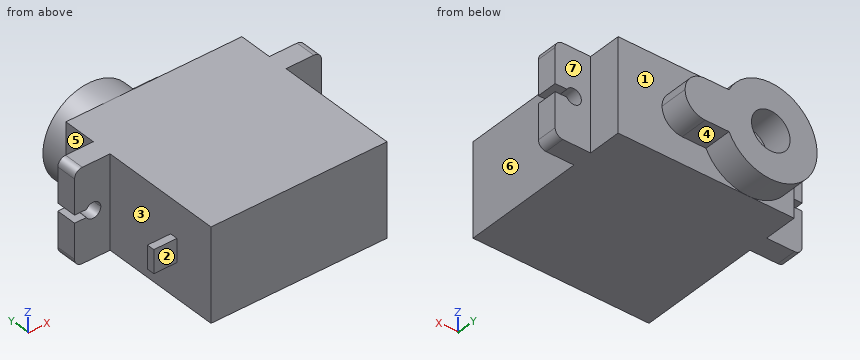
from build123d import *

# Parameters (mm, degrees)
SKETCH1_W                       = 22.8
SKETCH1_H                       = 12
BOSS_EXTRUDE1_DEPTH             = 16
SKETCH2_W                       = 32
SKETCH2_H                       = 12
BOSS_EXTRUDE2_DEPTH             = 2.65
BOSS_EXTRUDE3_REACH             = 25.409
SKETCH3_W                       = 22.8
SKETCH3_H                       = 23
BOSS_EXTRUDE3_DIRECTION_2_REACH = 25.409
CUT_EXTRUDE1_REACH              = 27.295
FILLET1_R                       = 1
SKETCH5_R                       = 6
BOSS_EXTRUDE4_DEPTH             = 3.65
BOSS_EXTRUDE5_DEPTH             = 3.65
SKETCH7_R                       = 2.5
CUT_EXTRUDE2_DEPTH              = 3.65
SKETCH8_W                       = 3
SKETCH8_H                       = 1
BOSS_EXTRUDE6_DEPTH             = 3


with BuildPart() as part:
    # Sketch1 → Boss-Extrude1 (new body)
    with BuildSketch(Plane(origin=(0, 0, 0), x_dir=(1, 0, 0), z_dir=(0, 1, 0))):
        Rectangle(SKETCH1_W, SKETCH1_H)
    extrude(amount=-BOSS_EXTRUDE1_DEPTH)

    # Sketch2 → Boss-Extrude2 (add)
    with BuildSketch(Plane(origin=(0, 0, 0), x_dir=(1, 0, 0), z_dir=(0, 1, 0))):
        Rectangle(SKETCH2_W, SKETCH2_H)
    extrude(amount=BOSS_EXTRUDE2_DEPTH)

    # Boss-Extrude3: up to this face of the body (flat: up to its plane)
    boss_extrude3_end = Plane(part.part.faces().sort_by_distance((0, -6.241192171, 6))[0])
    # Sketch3 → Boss-Extrude3 (add, up to the picked face)
    with BuildSketch(Plane.XY, mode=Mode.PRIVATE) as boss_extrude3_sk1:
        with Locations((0, -4.5)):
            Rectangle(SKETCH3_W, SKETCH3_H)
    boss_extrude3_tool1 = split(extrude(boss_extrude3_sk1.sketch, amount=BOSS_EXTRUDE3_REACH, mode=Mode.PRIVATE), bisect_by=boss_extrude3_end, keep=Keep.BOTH, mode=Mode.PRIVATE)
    add(boss_extrude3_tool1.solids().sort_by(Axis((0, -4.5, 0), (0, 0, 1)))[0])

    # Boss-Extrude3 direction 2: up to this face of the body (flat: up to its plane)
    boss_extrude3_direction_2_end = Plane(part.part.faces().sort_by_distance((0, -6.241192171, -6))[0])
    # Sketch3 → Boss-Extrude3 direction 2 (add, up to the picked face)
    with BuildSketch(Plane.XY, mode=Mode.PRIVATE) as boss_extrude3_direction_2_sk1:
        with Locations((0, -4.5)):
            Rectangle(SKETCH3_W, SKETCH3_H)
    boss_extrude3_direction_2_tool1 = split(extrude(boss_extrude3_direction_2_sk1.sketch, amount=-BOSS_EXTRUDE3_DIRECTION_2_REACH, mode=Mode.PRIVATE), bisect_by=boss_extrude3_direction_2_end, keep=Keep.BOTH, mode=Mode.PRIVATE)
    add(boss_extrude3_direction_2_tool1.solids().sort_by(Axis((0, -4.5, 0), (0, 0, -1)))[0])

    # Sketch4 → Cut-Extrude1 (cut, up to next)
    with BuildSketch(Plane(origin=(0, 2.65, 0), x_dir=(1, 0, 0), z_dir=(0, 1, 0)), mode=Mode.PRIVATE) as cut_extrude1_sk1:
        with BuildLine():
            ThreePointArc((14.6, 0), (14.565925826, 0.258819045), (14.466025404, 0.5))
            Line((14.466025404, 0.5), (13.6, 0.5))
            Line((13.6, 0.5), (13.6, -0.5))
            Line((13.6, -0.5), (14.466025404, -0.5))
            ThreePointArc((14.466025404, -0.5), (14.565925826, -0.258819045), (14.6, 0))
        make_face()
    cut_extrude1_tool1 = extrude(cut_extrude1_sk1.sketch, amount=-CUT_EXTRUDE1_REACH, mode=Mode.PRIVATE) & part.part
    # Sketch4 → Cut-Extrude1 (cut, up to next)
    with BuildSketch(Plane(origin=(0, 2.65, 0), x_dir=(1, 0, 0), z_dir=(0, 1, 0)), mode=Mode.PRIVATE) as cut_extrude1_sk2:
        with BuildLine():
            Line((13.6, 0.5), (14.466025404, 0.5))
            ThreePointArc((14.466025404, 0.5), (12.6, 0), (14.466025404, -0.5))
            Line((14.466025404, -0.5), (13.6, -0.5))
            Line((13.6, -0.5), (13.6, 0.5))
        make_face()
    cut_extrude1_tool2 = extrude(cut_extrude1_sk2.sketch, amount=-CUT_EXTRUDE1_REACH, mode=Mode.PRIVATE) & part.part
    # Sketch4 → Cut-Extrude1 (cut, up to next)
    with BuildSketch(Plane(origin=(0, 2.65, 0), x_dir=(1, 0, 0), z_dir=(0, 1, 0)), mode=Mode.PRIVATE) as cut_extrude1_sk3:
        with BuildLine():
            ThreePointArc((14.6, 0), (14.565925826, 0.258819045), (14.466025404, 0.5))
            Line((14.466025404, 0.5), (13.6, 0.5))
            Line((13.6, 0.5), (13.6, -0.5))
            Line((13.6, -0.5), (14.466025404, -0.5))
            ThreePointArc((14.466025404, -0.5), (14.565925826, -0.258819045), (14.6, 0))
        make_face()
    cut_extrude1_tool3 = extrude(cut_extrude1_sk3.sketch, amount=-CUT_EXTRUDE1_REACH, mode=Mode.PRIVATE) & part.part
    # Sketch4 → Cut-Extrude1 (cut, up to next)
    with BuildSketch(Plane(origin=(0, 2.65, 0), x_dir=(1, 0, 0), z_dir=(0, 1, 0)), mode=Mode.PRIVATE) as cut_extrude1_sk4:
        with BuildLine():
            Line((13.6, 0.5), (14.466025404, 0.5))
            ThreePointArc((14.466025404, 0.5), (12.6, 0), (14.466025404, -0.5))
            Line((14.466025404, -0.5), (13.6, -0.5))
            Line((13.6, -0.5), (13.6, 0.5))
        make_face()
    cut_extrude1_tool4 = extrude(cut_extrude1_sk4.sketch, amount=-CUT_EXTRUDE1_REACH, mode=Mode.PRIVATE) & part.part
    # Sketch4 → Cut-Extrude1 (cut, up to next)
    with BuildSketch(Plane(origin=(0, 2.65, 0), x_dir=(1, 0, 0), z_dir=(0, 1, 0)), mode=Mode.PRIVATE) as cut_extrude1_sk5:
        with BuildLine():
            Line((16, -0.5), (16, 0.5))
            Line((16, 0.5), (14.466025404, 0.5))
            ThreePointArc((14.466025404, 0.5), (14.565925826, 0.258819045), (14.6, 0))
            ThreePointArc((14.6, 0), (14.565925826, -0.258819045), (14.466025404, -0.5))
            Line((14.466025404, -0.5), (16, -0.5))
        make_face()
    cut_extrude1_tool5 = extrude(cut_extrude1_sk5.sketch, amount=-CUT_EXTRUDE1_REACH, mode=Mode.PRIVATE) & part.part
    # Sketch4 → Cut-Extrude1 (cut, up to next)
    with BuildSketch(Plane(origin=(0, 2.65, 0), x_dir=(1, 0, 0), z_dir=(0, 1, 0)), mode=Mode.PRIVATE) as cut_extrude1_sk6:
        with BuildLine():
            Line((-14.466025404, 0.5), (-16, 0.5))
            Line((-16, 0.5), (-16, -0.5))
            Line((-16, -0.5), (-14.466025404, -0.5))
            ThreePointArc((-14.466025404, -0.5), (-14.6, 0), (-14.466025404, 0.5))
        make_face()
    cut_extrude1_tool6 = extrude(cut_extrude1_sk6.sketch, amount=-CUT_EXTRUDE1_REACH, mode=Mode.PRIVATE) & part.part
    # Sketch4 → Cut-Extrude1 (cut, up to next)
    with BuildSketch(Plane(origin=(0, 2.65, 0), x_dir=(1, 0, 0), z_dir=(0, 1, 0)), mode=Mode.PRIVATE) as cut_extrude1_sk7:
        with BuildLine():
            ThreePointArc((-12.6, 0), (-13.341180955, 0.965925826), (-14.466025404, 0.5))
            Line((-14.466025404, 0.5), (-13.6, 0.5))
            Line((-13.6, 0.5), (-13.6, -0.5))
            Line((-13.6, -0.5), (-14.466025404, -0.5))
            ThreePointArc((-14.466025404, -0.5), (-13.341180955, -0.965925826), (-12.6, 0))
        make_face()
    cut_extrude1_tool7 = extrude(cut_extrude1_sk7.sketch, amount=-CUT_EXTRUDE1_REACH, mode=Mode.PRIVATE) & part.part
    # Sketch4 → Cut-Extrude1 (cut, up to next)
    with BuildSketch(Plane(origin=(0, 2.65, 0), x_dir=(1, 0, 0), z_dir=(0, 1, 0)), mode=Mode.PRIVATE) as cut_extrude1_sk8:
        with BuildLine():
            Line((-13.6, 0.5), (-14.466025404, 0.5))
            ThreePointArc((-14.466025404, 0.5), (-14.6, 0), (-14.466025404, -0.5))
            Line((-14.466025404, -0.5), (-13.6, -0.5))
            Line((-13.6, -0.5), (-13.6, 0.5))
        make_face()
    cut_extrude1_tool8 = extrude(cut_extrude1_sk8.sketch, amount=-CUT_EXTRUDE1_REACH, mode=Mode.PRIVATE) & part.part
    # Sketch4 → Cut-Extrude1 (cut, up to next)
    with BuildSketch(Plane(origin=(0, 2.65, 0), x_dir=(1, 0, 0), z_dir=(0, 1, 0)), mode=Mode.PRIVATE) as cut_extrude1_sk9:
        with BuildLine():
            ThreePointArc((-12.6, 0), (-13.341180955, 0.965925826), (-14.466025404, 0.5))
            Line((-14.466025404, 0.5), (-13.6, 0.5))
            Line((-13.6, 0.5), (-13.6, -0.5))
            Line((-13.6, -0.5), (-14.466025404, -0.5))
            ThreePointArc((-14.466025404, -0.5), (-13.341180955, -0.965925826), (-12.6, 0))
        make_face()
    cut_extrude1_tool9 = extrude(cut_extrude1_sk9.sketch, amount=-CUT_EXTRUDE1_REACH, mode=Mode.PRIVATE) & part.part
    # Sketch4 → Cut-Extrude1 (cut, up to next)
    with BuildSketch(Plane(origin=(0, 2.65, 0), x_dir=(1, 0, 0), z_dir=(0, 1, 0)), mode=Mode.PRIVATE) as cut_extrude1_sk10:
        with BuildLine():
            Line((-13.6, 0.5), (-14.466025404, 0.5))
            ThreePointArc((-14.466025404, 0.5), (-14.6, 0), (-14.466025404, -0.5))
            Line((-14.466025404, -0.5), (-13.6, -0.5))
            Line((-13.6, -0.5), (-13.6, 0.5))
        make_face()
    cut_extrude1_tool10 = extrude(cut_extrude1_sk10.sketch, amount=-CUT_EXTRUDE1_REACH, mode=Mode.PRIVATE) & part.part
    add(cut_extrude1_tool1.solids().sort_by_distance((14.079122, 2.65, 0))[0], mode=Mode.SUBTRACT)
    add(cut_extrude1_tool2.solids().sort_by_distance((13.390235, 2.65, 0))[0], mode=Mode.SUBTRACT)
    add(cut_extrude1_tool3.solids().sort_by_distance((14.079122, 2.65, 0))[0], mode=Mode.SUBTRACT)
    add(cut_extrude1_tool4.solids().sort_by_distance((13.390235, 2.65, 0))[0], mode=Mode.SUBTRACT)
    add(cut_extrude1_tool5.solids().sort_by_distance((15.277765, 2.65, 0))[0], mode=Mode.SUBTRACT)
    add(cut_extrude1_tool6.solids().sort_by_distance((-15.277765, 2.65, 0))[0], mode=Mode.SUBTRACT)
    add(cut_extrude1_tool7.solids().sort_by_distance((-13.390235, 2.65, 0))[0], mode=Mode.SUBTRACT)
    add(cut_extrude1_tool8.solids().sort_by_distance((-14.079122, 2.65, 0))[0], mode=Mode.SUBTRACT)
    add(cut_extrude1_tool9.solids().sort_by_distance((-13.390235, 2.65, 0))[0], mode=Mode.SUBTRACT)
    add(cut_extrude1_tool10.solids().sort_by_distance((-14.079122, 2.65, 0))[0], mode=Mode.SUBTRACT)

    # Fillet1
    fillet1_edges = [part.edges().sort_by_distance(p)[0] for p in [
        (16, 1.325, 6),
        (16, 1.325, -6),
        (-16, 1.325, -6),
        (-16, 1.325, 6),
    ]]
    fillet(fillet1_edges, radius=FILLET1_R)

    # Sketch5 → Boss-Extrude4 (add)
    with BuildSketch(Plane(origin=(0, 7, 0), x_dir=(1, 0, 0), z_dir=(0, 1, 0))):
        with Locations(Location((-5.4, 0, 0), (0, 0, 270))):
            Circle(SKETCH5_R)
    extrude(amount=BOSS_EXTRUDE4_DEPTH)

    # Sketch6 → Boss-Extrude5 (add)
    with BuildSketch(Plane(origin=(0, 7, 0), x_dir=(1, 0, 0), z_dir=(0, 1, 0))):
        with BuildLine():
            Line((0.007402334, -2.6), (3.1, -2.6))
            ThreePointArc((3.1, -2.6), (1.487245955, -2.039368625), (0.57, -0.599249531))
            ThreePointArc((0.57, -0.599249531), (0.375990961, -1.624170072), (0.007402334, -2.6))
        make_face()
        with BuildLine():
            ThreePointArc((0.57, 0.599249531), (1.487245955, 2.039368625), (3.1, 2.6))
            Line((3.1, 2.6), (0.007402334, 2.6))
            ThreePointArc((0.007402334, 2.6), (0.375990961, 1.624170072), (0.57, 0.599249531))
        make_face()
        with BuildLine():
            ThreePointArc((5.7, 0), (4.938477631, 1.838477631), (3.1, 2.6))
            ThreePointArc((3.1, 2.6), (1.487245955, 2.039368625), (0.57, 0.599249531))
            ThreePointArc((0.57, 0.599249531), (0.592495307, 0.3), (0.6, 0))
            ThreePointArc((0.6, 0), (0.592495307, -0.3), (0.57, -0.599249531))
            ThreePointArc((0.57, -0.599249531), (1.487245955, -2.039368625), (3.1, -2.6))
            ThreePointArc((3.1, -2.6), (4.938477631, -1.838477631), (5.7, 0))
        make_face()
        with BuildLine():
            ThreePointArc((0.6, 0), (0.592495307, 0.3), (0.57, 0.599249531))
            ThreePointArc((0.57, 0.599249531), (0.5, 0), (0.57, -0.599249531))
            ThreePointArc((0.57, -0.599249531), (0.592495307, -0.3), (0.6, 0))
        make_face()
    extrude(amount=BOSS_EXTRUDE5_DEPTH)

    # Sketch7 → Cut-Extrude2 (cut)
    with BuildSketch(Plane(origin=(0, 10.65, 0), x_dir=(1, 0, 0), z_dir=(0, 1, 0))):
        with Locations(Location((-5.4, 0, 0), (0, 0, 270))):
            Circle(SKETCH7_R)
    extrude(amount=-CUT_EXTRUDE2_DEPTH, mode=Mode.SUBTRACT)

    # Sketch8 → Boss-Extrude6 (add)
    with BuildSketch(Plane.ZY.offset(11.4)):
        with Locations((0, -10.1)):
            Rectangle(SKETCH8_W, SKETCH8_H)
    extrude(amount=BOSS_EXTRUDE6_DEPTH)


solid = part.part
Geometry check sheet. Reference: the model listing, model coordinates, mm. Face numbers are marked on the shaded views. A direction names the side the tool comes from. Round coordinates to 2 decimals unless told otherwise and drop trailing zeros. Order: outer loops, then holes, each group sorted by start corner. A loop starts at its lowest first (then second) coordinate and runs counter-clockwise, first axis right, second up. Notation, with made-up numbers: (10, 61) - (40, 61) arc R32 ccw to (40, 93) - close; hole circle Ø6 at (69, -12). An arc over 180 degrees is marked (long way). One line per question, with ' | ' between items. Start each with the question number.
(1) Depth check by flat-ended pin: pin 1 Ø3 at (x, z) = (-5.4, 0) entering from +Y; pin 2 Ø3.5 at (x, z) = (13.5, 1.5) entering from +Y; pin 3 Ø1.5 at (y, z) = (3.5, -2) entering from -X. Enter the tip coordinate at first touch or a pass-through.
(2) Sectioned sample at D-D on x = 4. Record the cut outline in (y, z).
(3) Access from +Z, -Z, +X, -X, +Y, -Y to the whole of each face (thin tool, end or side, straight path). Record for the marked faces 4, 5, 6 and 7.
(4) Sectioned sample at B-B on y = 9.25. Record the cut outline in (x, z), and give its area (3 significant figures).
(5) Sectioned sample at A-A on x = 13.6. Record the cut outline in (y, z).
(6) Sectioned sample at C-C on z = -3. Record the cut outline in (x, y).
(7) Thickness scan on L1, parallel to X at y = 9.25, z = 0; L2, parallel to Y at x = -14, z = 1; L3, parallel to Y at x = 2.5, z = 2.75. Record the ranges inside material, lowest first. Write a range as [from, to].
(8) Release check for a two-part mould opening along Y. For the marked faces 1, 2 and 3 record: released by +Y, released by -Y, zero draft, split by the parting line, or undercut.
Conclusion:
1) pin 1: stops at y = 7 | pin 2: stops at y = 2.65 | pin 3: stops at x = -11.4
2) outline: (-16, -6) - (7, -6) - (7, -2.44) - (10.65, -2.44) - (10.65, 2.44) - (7, 2.44) - (7, 6) - (-16, 6) - close
3) face 4: -Z, +X, +Y | face 5: +Z, -Z, -X, +Y | face 6: +Z, -Z, +X, -Y | face 7: +Z, -Z, +X, +Y
4) outline: (0.01, -2.6) - (3.1, -2.6) arc R2.6 ccw to (3.1, 2.6) - (0.01, 2.6) arc R6 ccw (long way) to start; hole circle Ø5 at (-5.4, 0) | area: 118 mm2
5) outline: (0, -6) - (2.65, -6) - (2.65, -1) - (0, -1) - close; (0, 1) - (2.65, 1) - (2.65, 6) - (0, 6) - close
6) outline: (-16, 0) - (-11.4, 0) - (-11.4, -16) - (11.4, -16) - (11.4, 0) - (16, 0) - (16, 2.65) - (11.4, 2.65) - (11.4, 7) - (-0.2, 7) - (-0.2, 10.65) - (-10.6, 10.65) - (-10.6, 7) - (-11.4, 7) - (-11.4, 2.65) - (-16, 2.65) - close
7) L1: x = [-11.4, -7.9], [-2.9, 5.7] | L2: y = [-10.6, -9.6], [0, 2.65] | L3: y = [-16, 7]
8) face 1: released by +Y | face 2: released by -Y | face 3: undercut
